```python
from build123d import *

# Parameters (mm, degrees)
F1_DEPTH = 2
F2_W     = 10
F2_H     = 10
F3_DEPTH = 3
F4_R     = 1.5
F4_R_2   = 1.4
F5_DEPTH = 5


with BuildPart() as f1:
    # F0 (on Top) → F1 (new body)
    with BuildSketch(Plane.XY):
        Polygon((-52.435034, 59.411056), (-62.435034, 59.411056), (-62.435034, -2.588944), (-28.435034, -2.588944), (-28.435034, -9.588944), (7.564966, -9.588944), (7.564966, 32.411056), (-28.435034, 32.411056), (-28.435034, 4.411056), (-40.435034, 4.411056), (-40.435034, 7.411056), (-52.435034, 7.411056), align=None)
    extrude(amount=F1_DEPTH)

    # F2 (on face) → F3 (join)
    with BuildSketch(Plane(origin=(0, 0, 0), x_dir=(1, 0, 0), z_dir=(0, 0, -1))):
        with Locations((-57.435034, -54.411056)):
            Rectangle(F2_W, F2_H)
        with Locations((-57.435034, -2.411056)):
            Rectangle(F2_W, F2_H)
        with Locations((2.564966, -2.411056)):
            Rectangle(F2_W, F2_H)
    extrude(amount=F3_DEPTH)

    # F4 (on face) → F5 (cut)
    with BuildSketch(Plane.XY.offset(2)):
        with Locations((-57.435034, 54.411056)):
            Circle(F4_R)
        with Locations((-57.435034, 2.411056)):
            Circle(F4_R)
        with Locations((2.564966, 2.411056)):
            Circle(F4_R)
        with Locations((-6.935034, 26.911056)):
            Circle(F4_R_2)
        with Locations((-22.935034, -4.088944)):
            Circle(F4_R_2)
    extrude(amount=-F5_DEPTH, mode=Mode.SUBTRACT)


solid = f1.part
```
The model under review builds one solid part; all positions refer to its coordinate system, in mm. A direction names the side the tool comes from. Round coordinates to 2 decimals unless told otherwise and drop trailing zeros. Write each loop counter-clockwise with the first axis right and the second up, starting at its lowest first coordinate (ties: lowest second). Pieces come first, ordered by that corner, then holes. Notation, with made-up numbers: (2, 23.25) - (13, 23.25) arc R26 ccw to (13, 41.25) - close; hole circle Ø4 at (-22, -40). An arc over 180 degrees is marked (long way). Use one line per item in the form item = value.
Q1. For line 1 (X direction, y = 0.5, z = -2.05); line 2 (X direction, y = 2, z = 0.9); line 3 (Y direction, x = -14.5, z = 0.15), list the stretches that pass through material, from the lowest coordinate up. Write a range as [from, to].
Answer key:
line_1 = [-62.44, -52.44], [-2.44, 7.56]
line_2 = [-62.44, -58.88], [-55.99, 1.12], [4.01, 7.56]
line_3 = [-9.59, 32.41]
Q2. Consider section A-A (y = 15.5). State the section outline as (x, z) points.
Answer key:
outline = (-62.44, 0) - (-52.44, 0) - (-52.44, 2) - (-62.44, 2) - close; (-28.44, 0) - (7.56, 0) - (7.56, 2) - (-28.44, 2) - close
Q3. Insertion check: pin 1 Ø2 at (y, z) = (-5.5, 1) entering from -X; pin 2 Ø2.5 at (x, y) = (2.56, 2.41) entering from -Z; pin 3 Ø3.5 at (x, y) = (-6.94, 26.91) entering from -Z; pin 4 Ø2 at (x, z) = (-0.5, -2) entering from +Y. Each pin has a flat end and moves straight along its axis. Give the tip position at first contact, or say it passes through.
Answer key:
pin_1 = -28.44
pin_2 = through
pin_3 = 0
pin_4 = 7.41
Q4. Consider section C-C (y = -1.5). State the section outline as (x, z) points, and give its area (3 significant figures).
Answer key:
outline = (-62.44, -3) - (-52.44, -3) - (-52.44, 0) - (-2.44, 0) - (-2.44, -3) - (7.56, -3) - (7.56, 2) - (-62.44, 2) - close
area = 200 mm2
Q5. Draft analysis for pull direction Y (two halves, no side actions). For faces 1 (the flat face through (1, 1, -3)), 2 (the cylindrical face through (2.24, 0.947, -0.465)), 3 (the flat face through (-10, 32.411, 1)), state which applies: +Y half, -Y half, draft (parallel to the pull), parting line (faces both ways), or undercut.
Answer key:
face_1 = draft
face_2 = undercut
face_3 = +Y half
Q6. Consider section D-D (x = -30.5). State the section outline as (y, z) points, and give its area (3 significant figures).
Answer key:
outline = (-2.59, 0) - (4.41, 0) - (4.41, 2) - (-2.59, 2) - close
area = 14.0 mm2
Q7. Tool access review of faces 4 (the flat face through (2, 7.411, -1)), 5 (the flat face through (2, -2.589, -1)), 6 (the flat face through (-40.435, 6, 1)): name each direction out of +Z, -Z, +X, -X, +Y, -Y from which nothing blocks a thin tool from reaching the whole face with its end or side.
Answer key:
face_4 = -Z, +X, -X, +Y
face_5 = -Z, +X, -X, -Y
face_6 = +Z, -Z, +Y
Q8. Consider section B-B (z = -1.9). State the section outline as (x, y) points, and give its area (3 significant figures).
Answer key:
outline = (-62.44, -2.59) - (-52.44, -2.59) - (-52.44, 7.41) - (-62.44, 7.41) - close; (-62.44, 49.41) - (-52.44, 49.41) - (-52.44, 59.41) - (-62.44, 59.41) - close; (-2.44, -2.59) - (7.56, -2.59) - (7.56, 7.41) - (-2.44, 7.41) - close; hole circle Ø3 at (-57.44, 2.41); hole circle Ø3 at (-57.44, 54.41); hole circle Ø3 at (2.56, 2.41)
area = 279 mm2
